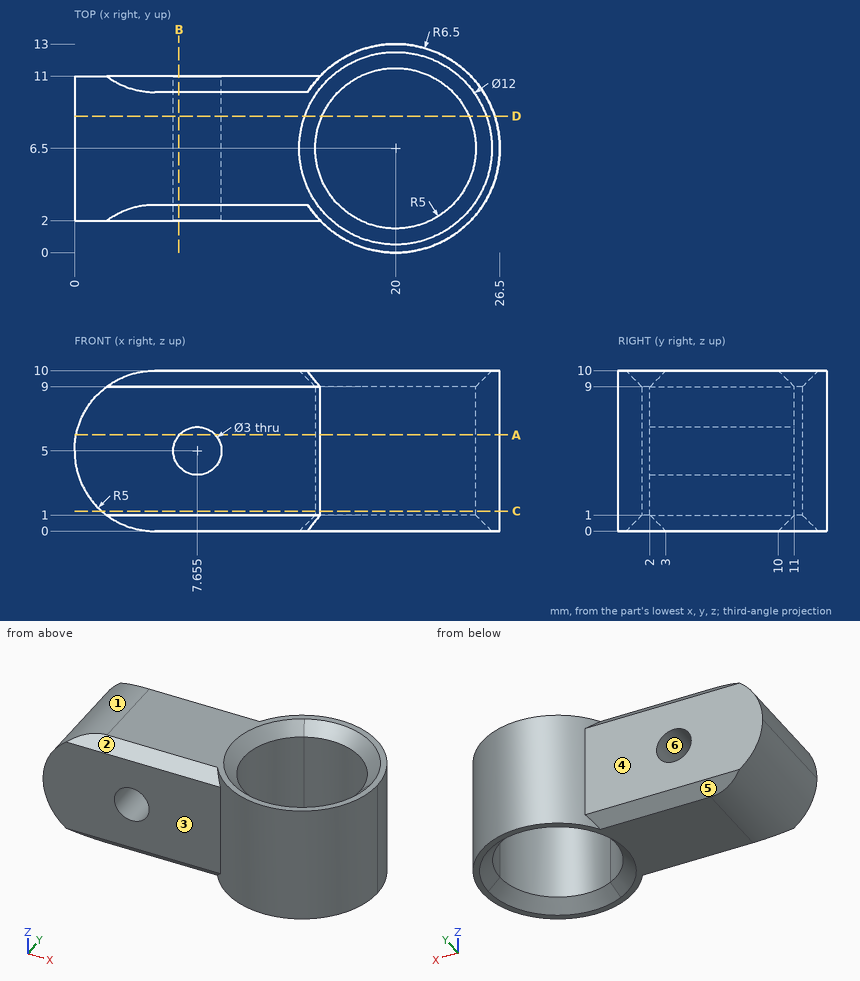
Part print with two shaded views. Sizes in mm from the minimum x, y, z corner. A direction names the side the tool comes from. Coordinates: 2 decimals unless noted, no trailing zeros. Loops run counter-clockwise (first coordinate to the right, second up) from the corner with the lowest first, then second, coordinate; pieces in that order, holes last. Notation, with made-up numbers: (-37.5, 35) -> (18.5, 35) arc R24 ccw to (18.5, 63) -> close; hole circle Ø3 at (66, 1.5). An arc over 180 degrees is marked (long way). Answer as a JSON object with one key per item and string values.
Q1. Cut at C-C (z = 1.25). List the corners of the cut face in (x, y), and give its area (3 significant figures).
Report:
{"outline": "(1.69, 2) -> (15.31, 2) arc R6.5 ccw (long way) to (15.31, 11) -> (1.69, 11) -> close; hole circle Ø10 at (20, 6.5)", "area": "166 mm2"}
Q2. Cut at B-B (x = 6.5). List the corners of the cut face in (y, z).
Report:
{"outline": "(2, 1) -> (3, 0) -> (10, 0) -> (11, 1) -> (11, 4.04) -> (2, 4.04) -> close; (2, 5.96) -> (11, 5.96) -> (11, 9) -> (10, 10) -> (3, 10) -> (2, 9) -> close"}
Q3. Cut at D-D (y = 8.5). State how many separate pieces and enclosed holes the cut face has, and give its area (3 significant figures).
Report:
{"separate pieces": "2", "enclosed holes": "1", "area": "150 mm2"}
Q4. Pull direction Z, two halves, no side cores. Call the marked faces 4, 5 and 6: released by +Z, released by -Z, zero draft, split by the parting line, or undercut.
Report:
{"face 4": "zero draft", "face 5": "released by -Z", "face 6": "undercut"}
Q5. Cut at A-A (z = 6). List the corners of the cut face in (x, y), and give its area (3 significant figures).
Report:
{"outline": "(0.1, 2) -> (6.54, 2) -> (6.54, 11) -> (0.1, 11) -> close; (8.77, 2) -> (15.31, 2) arc R6.5 ccw (long way) to (15.31, 11) -> (8.77, 11) -> close; hole circle Ø10 at (20, 6.5)", "area": "160 mm2"}
Q6. Probe probe 1 along Y at (x, z) = (11.5, 2); probe 2 along Y at (x, z) = (23.5, 2.5); probe 3 along X at (y, z) = (2.25, 7) (1 decimal). List the from-to ranges inside material, lowest first.
Report:
{"probe 1": "y = 2 to 11", "probe 2": "y = 1.02 to 2.93, 10.07 to 11.98", "probe 3": "x = 0.4 to 17.4, 22.6 to 24.9"}
Q7. 3-axis set-ups, long thin cutter, end or side, ignore diameter. For the marked faces 1, 2 and 3: which of +Z, -Z, +X, -X, +Y, -Y reach the whole face in a straight line?
Report:
{"face 1": "+Z, -X, +Y, -Y", "face 2": "+Z, -X, -Y", "face 3": "+Z, -Z, -X, -Y"}
Q8. Flat gauge pins, fed straight in: P1, Ø4, axis at x = 5, z = 6, coming from the -Y side; P2, Ø2, axis at x = 21.5, z = 5.5, coming from the +Y side; P3, Ø3.5, axis at x = 7.65, z = 5, coming from the +Y side. Where does each tip first touch, or does it go through?
Report:
{"P1": "stops at y = 2", "P2": "stops at y = 12.98", "P3": "stops at y = 11"}
